from build123d import *

# Parameters (mm, degrees)
IZIM1_R                          = 3.5
IZIM1_W                          = 61
IZIM1_H                          = 46
Y_KSEKLIK_EKSTR_ZYON1_DEPTH      = 5
Y_KSEKLIK_EKSTR_ZYON2_DEPTH      = 5
Y_KSEKLIK_EKSTR_ZYON2_DEPTH_BACK = 5
PAH1_SIZE                        = 2
PAH2_SIZE                        = 2
IZIM5_R                          = 1.5
KES_EKSTR_ZYON1_DEPTH            = 10


with BuildPart() as part:
    # Çizim1 → Yükseklik-Ekstrüzyon1 (new body)
    with BuildSketch(Plane.XY):
        Polygon((-75, 70), (-75, 110), (-35, 70), (35, 70), (75, 110), (75, 70), (75, -20), (45, -50), (-45, -50), (-75, -20), align=None)
        with Locations((0, 25)):
            Circle(IZIM1_R, mode=Mode.SUBTRACT)
        with Locations((0, -15)):
            Rectangle(IZIM1_W, IZIM1_H, mode=Mode.SUBTRACT)
        with BuildLine():
            ThreePointArc((-26, 37), (-35.043252773, 47.813379198), (-49, 45.833783979))
            ThreePointArc((-49, 45.833783979), (-40.097413612, 34.654160049), (-26, 37))
        make_face(mode=Mode.SUBTRACT)
        with BuildLine():
            ThreePointArc((26, 37), (40.097413612, 34.654160049), (49, 45.833783979))
            ThreePointArc((49, 45.833783979), (35.043252773, 47.813379198), (26, 37))
        make_face(mode=Mode.SUBTRACT)
    extrude(amount=Y_KSEKLIK_EKSTR_ZYON1_DEPTH)

    # Çizim3 → Yükseklik-Ekstrüzyon2 (add, two sides: drawn at the far end of the back side and taken through both)
    with BuildSketch(Plane.XY.offset(5).offset(-Y_KSEKLIK_EKSTR_ZYON2_DEPTH_BACK)):
        with BuildLine():
            ThreePointArc((-26, 37), (-40.097413612, 34.654160049), (-49, 45.833783979))
            ThreePointArc((-49, 45.833783979), (-35.043252773, 47.813379198), (-26, 37))
        make_face()
        with BuildLine():
            ThreePointArc((26, 37), (35.043252773, 47.813379198), (49, 45.833783979))
            ThreePointArc((49, 45.833783979), (40.097413612, 34.654160049), (26, 37))
        make_face()
    extrude(amount=Y_KSEKLIK_EKSTR_ZYON2_DEPTH + Y_KSEKLIK_EKSTR_ZYON2_DEPTH_BACK)

    # Pah1
    pah1_edges = [part.edges().sort_by_distance(p)[0] for p in [
        (-35.043252773, 47.813379198, 10),
        (-40.097413612, 34.654160049, 10),
        (40.097413612, 34.654160049, 10),
        (35.043252773, 47.813379198, 10),
    ]]
    chamfer(pah1_edges, length=PAH1_SIZE)

    # Pah2
    pah2_edges = [part.edges().sort_by_distance(p)[0] for p in [
        (30.5, -15, 5),
        (0, 8, 5),
        (-30.5, -15, 5),
        (0, -38, 5),
    ]]
    chamfer(pah2_edges, length=PAH2_SIZE)

    # Çizim5 → Kes-Ekstrüzyon1 (cut)
    with BuildSketch(Plane.XY.offset(5)):
        with Locations((-65, 80)):
            Circle(IZIM5_R)
        with Locations((-52.5, -27.5)):
            Circle(IZIM5_R)
        with Locations(Location((52.5, -27.5, 0), (0, 0, 180))):
            Circle(IZIM5_R)
        with Locations(Location((65, 80, 0), (0, 0, 180))):
            Circle(IZIM5_R)
    extrude(amount=-KES_EKSTR_ZYON1_DEPTH, mode=Mode.SUBTRACT)


solid = part.part
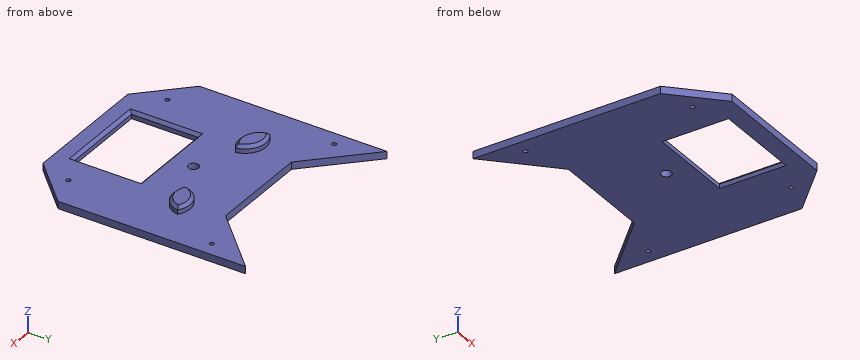
Read the model definition and answer for the solid it produces. Units are mm, in the model's axes. Give positions to 0.01 mm unless a question says otherwise; leave off trailing zeros. Write each loop counter-clockwise with the first axis right and the second up, starting at its lowest first coordinate (ties: lowest second). Pieces come first, ordered by that corner, then holes. Notation, with made-up numbers: (38.5, -13.5) -> (45.5, -13.5) arc R29 cw to (45.5, 21.5) -> close; hole circle Ø1 at (-10, -35). An arc over 180 degrees is marked (long way). Answer as a JSON object with one key per item and string values. Group by question number.
1) Find section A-A (y = 98). Write down the section's boundary in (x, z), and give its area (3 significant figures).
2) Each of these flat-tipped pins is pushed along its axis until it touches: P1, Ø10, axis at x = -42, y = -21, coming from the +Z side; P2, Ø1.5, axis at x = 9, z = 3.5, coming from the +Y side; P3, Ø0.9, axis at y = -25, z = 1.5, coming from the +X side. Where does it stop, or does it pass through?
3) Find section B-B (x = 0). Write down the section's boundary in (y, z), and give its area (3 significant figures).
4) Find section D-D (x = 57). Write down the section's boundary in (y, z).
5) Consider L1, parallel to X at y = 80, z = 3.95; L2, parallel to Y at x = 25, z = 1.5; L3, parallel to X at y = -8, z = 0.5. Determine where each line is inside the solid, lowest interval first. Write a range as from..to.
6) Find section C-C (y = 25). Write down the section's boundary in (x, z), and give its area (3 significant figures).
Values follow:
{
 "1": {"outline": "(-75, 0) -> (-63, 0) -> (-63, 5) -> (-75, 5) -> close; (63, 0) -> (75, 0) -> (75, 5) -> (63, 5) -> close", "area": "120 mm2"},
 "2": {"P1": "stops at z = 5", "P2": "stops at y = 70", "P3": "stops at x = 70.45"},
 "3": {"outline": "(-50, 0) -> (-38, 0) -> (-38, 3) -> (-40, 5) -> (-50, 5) -> close; (8, 0) -> (21.5, 0) -> (21.5, 5) -> (10, 5) -> (8, 3) -> close; (28.5, 0) -> (70, 0) -> (70, 5) -> (28.5, 5) -> close", "area": "331 mm2"},
 "4": {"outline": "(-38, 0) -> (92, 0) -> (92, 5) -> (-38, 5) -> close"},
 "5": {"L1": "x = -75..-66.5, -63.5..-45, 45..63.5, 66.5..75", "L2": "y = -50..-38, 8..70", "L3": "x = -75..-30.5, 30.5..75"},
 "6": {"outline": "(-75, 0) -> (-3.5, 0) -> (-3.5, 5) -> (-75, 5) -> close; (3.5, 0) -> (75, 0) -> (75, 5) -> (3.5, 5) -> close", "area": "715 mm2"}
}
